from build123d import *

# Parameters (mm, degrees)
SKETCH2_W          = 80
SKETCH2_H          = 40
SKETCH2_W_2        = 76
SKETCH2_H_2        = 36
CUT_EXTRUDE1_START = -10
SKETCH3_R          = 12.5
CUT_EXTRUDE1_DEPTH = 510
LPATTERN1_COUNT    = 16
LPATTERN1_PITCH    = 152
SKETCH4_R          = 6
CUT_EXTRUDE2_DEPTH = 10
LPATTERN2_COUNT    = 16
LPATTERN2_PITCH    = 152


with BuildPart() as part:
    # Sweep-Thin1: sweep along a path in Sketch1
    with BuildLine(Plane.XY) as sweep_thin1_path:
        Line((304, -1216), (-304, -1216))
        Line((-304, -1216), (-304, 1216))
        Line((-304, 1216), (304, 1216))
        Line((304, 1216), (304, -1216))
    # Sketch2 → Sweep-Thin1 (sweep)
    with BuildSketch(Plane(origin=(0, 0, 0), x_dir=(1, 0, 0), z_dir=(0, 1, 0))):
        with Locations((-264, 0)):
            Rectangle(SKETCH2_W, SKETCH2_H)
        with Locations((-264, 0)):
            Rectangle(SKETCH2_W_2, SKETCH2_H_2, mode=Mode.SUBTRACT)
    sweep(path=sweep_thin1_path.line, transition=Transition.RIGHT)

    # Sketch3 → Cut-Extrude1 (cut)
    with BuildSketch(Plane.ZY.offset(-224).offset(CUT_EXTRUDE1_START)):
        with Locations((0, 1142)):
            Circle(SKETCH3_R)
    cut_extrude1 = extrude(amount=CUT_EXTRUDE1_DEPTH, mode=Mode.SUBTRACT)

    # LPattern1: Cut-Extrude1 ×16
    with Locations(*[(0, -i * LPATTERN1_PITCH, 0) for i in range(1, LPATTERN1_COUNT)]):
        add(cut_extrude1, mode=Mode.SUBTRACT)

    # Sketch4 → Cut-Extrude2 (cut)
    with BuildSketch(Plane(origin=(304, 0, 0), x_dir=(0, 0, -1), z_dir=(1, 0, 0))):
        with Locations((0, 1142)):
            Circle(SKETCH4_R)
    cut_extrude2 = extrude(amount=-CUT_EXTRUDE2_DEPTH, mode=Mode.SUBTRACT)

    # LPattern2: Cut-Extrude2 ×16
    with Locations(*[(0, -i * LPATTERN2_PITCH, 0) for i in range(1, LPATTERN2_COUNT)]):
        add(cut_extrude2, mode=Mode.SUBTRACT)


solid = part.part
The listing builds one solid part. Answer for the finished solid, in the listing's coordinates (mm). A direction names the side the tool comes from. Give positions to 0.01 mm unless a question says otherwise; leave off trailing zeros. Order: outer loops, then holes, each group sorted by start corner. A loop starts at its lowest first (then second) coordinate and runs counter-clockwise, first axis right, second up. Notation, with made-up numbers: (-20, 10) - (2, 10) arc R8 cw to (2, 14) - close; hole circle Ø10 at (-11.75, 44). An arc over 180 degrees is marked (long way). Use one line per item in the form item = value.
1) The mould has two halves that part along Z. Classify faces 4 (the flat face through (-227, -96, 20)), 5 (the flat face through (304, -17, 0)), 6 (the flat face through (245, 96, 18)): released by +Z, released by -Z, zero draft, split by the parting line, or undercut.
Verdict:
face_4 = released by +Z
face_5 = zero draft
face_6 = undercut
2) This flat-tipped pin is pushed along its axis until it touches: pin 1 (7 mm diameter, centred on y = 382, z = 0, fed in from +X). Where does it stop, or does it pass through?
Verdict:
pin_1 = -302
3) For faces 1 (the flat face through (-304, 17, 0)), 2 (the flat face through (245, -96, -18)), 3 (the flat face through (224, -16, 0)), determine the directions among +Z, -Z, +X, -X, +Y, -Y from which every point of the face is accessible in a straight line to the end or side of a thin tool.
Verdict:
face_1 = +Z, -Z, -X, +Y, -Y
face_2 = none
face_3 = +Z, -Z
4) Find section B-B on x = 107.5. Determine the outline of the cut face in (y, z), and give its area (3 significant figures).
Verdict:
outline = (-1216, -20) - (-1136, -20) - (-1136, -12.34) arc R12.5 cw to (-1138, -12.5) - (-1138, -18) - (-1214, -18) - (-1214, 18) - (-1138, 18) - (-1138, 12.5) arc R12.5 cw to (-1136, 12.34) - (-1136, 20) - (-1216, 20) - close; (1136, -20) - (1216, -20) - (1216, 20) - (1136, 20) - (1136, 10.97) arc R12.5 cw to (1138, 11.84) - (1138, 18) - (1214, 18) - (1214, -18) - (1138, -18) - (1138, -11.84) arc R12.5 cw to (1136, -10.97) - close
area = 832 mm^2
5) Find section A-A on y = 627. Determine the outline of the cut face in (x, z), and give its area (3 significant figures).
Verdict:
outline = (-304, -20) - (-224, -20) - (-224, 20) - (-304, 20) - close; (224, -20) - (304, -20) - (304, 20) - (224, 20) - close; hole (-302, -18) - (-226, -18) - (-226, 18) - (-302, 18) - close; hole (226, -18) - (302, -18) - (302, 18) - (226, 18) - close
area = 928 mm^2
6) Consider probe 1 along X at (y, z) = (715, 10.5); probe 2 along Z at (x, y) = (-262.5, 628.5); probe 3 along Z at (x, y) = (224.8, 990). Determine where each line is inside the solid, lowest interval first. Write a range as [from, to].
Verdict:
probe_1 = [-304, -302], [-226, -224], [224, 226], [302, 304]
probe_2 = [-20, -18], [18, 20]
probe_3 = [-20, -12.5], [12.5, 20]
